```python
from build123d import *

# Parameters (mm, degrees)
F1_DEPTH    = 3
F3_DEPTH    = 5
F5_D        = 2
F5_DEPTH    = 2.001
F6_W        = 16.9
F6_H        = 5
F6_W_2      = 5
F7_DEPTH    = 4
F8_W        = 2
F8_H        = 3
F9_DEPTH    = 2.5
F11_DEPTH   = 2
F12_R       = 2
F13_SIZE2   = 1
F13_SIZE    = 0.2679491924
F14_SIZE2   = 2
F14_SIZE    = 0.5358983849
F14_2_SIZE2 = 2
F14_2_SIZE  = 0.5358983849
F15_SIZE2   = 1
F15_SIZE    = 0.5773502692
F16_W       = 15
F16_H       = 14
F17_DEPTH   = 8
F19_DEPTH   = 6
F21_D       = 2.5
F21_DEPTH   = 7.5
F21_TIP     = 0.7510757738


with BuildPart() as f1:
    # F0 (on Top) → F1 (new body, symmetric)
    with BuildSketch(Plane.XY):
        Polygon((19.45, 10), (0, 10), (-19.45, 10), (-19.45, -10), (19.45, -10), align=None)
    extrude(amount=F1_DEPTH, both=True)

    # F2 (on Front) → F3 (join, symmetric)
    with BuildSketch(Plane.XZ):
        Polygon((-8.45, 3.5893841543), (-16.45, 5), (-19.45, 5), (-19.45, 3), (-8.45, 3), align=None)
    extrude(amount=F3_DEPTH, both=True)

    # F5 (through all, one way)
    with BuildSketch(Plane(origin=(0, 0, 3), x_dir=(1, 0, 0), z_dir=(0, 0, -1))):
        with Locations((-8.45, -4), (-8.45, 4)):
            Circle(F5_D / 2)
    extrude(amount=-F5_DEPTH, mode=Mode.SUBTRACT)

    # F6 (on face) → F7 (join)
    with BuildSketch(Plane.XY.offset(3)):
        with Locations((-11, -7.5)):
            Rectangle(F6_W, F6_H)
        with Locations((-11, 7.5)):
            Rectangle(F6_W, F6_H)
        with Locations((16.95, 7.5)):
            Rectangle(F6_W_2, F6_H)
        with Locations((16.95, -7.5)):
            Rectangle(F6_W_2, F6_H)
    extrude(amount=F7_DEPTH)

    # F8 (on face) → F9 (join)
    with BuildSketch(Plane.XY.offset(3)):
        with Locations((3.45, 6.5)):
            Rectangle(F8_W, F8_H)
        with Locations((3.45, -6.5)):
            Rectangle(F8_W, F8_H)
    extrude(amount=F9_DEPTH)

    # F10 (on face) → F11 (join)
    with BuildSketch(Plane.XY.offset(3)):
        Polygon((19.45, -5), (19.45, 5), (14.45, 5), (14.45, 2), (8.45, 2), (8.45, -2), (14.45, -2), (14.45, -5), align=None)
    extrude(amount=F11_DEPTH)

    # F12
    f12_edges = [f1.edges().sort_by_distance(p)[0] for p in [
        (14.45, -2, 4),
        (14.45, 2, 4),
    ]]
    fillet(f12_edges, radius=F12_R)

    # F13
    f13_edges = [f1.edges().sort_by_distance(p)[0] for p in [
        (8.45, 0, 5),
    ]]
    f13_side = f1.faces().sort_by_distance((15.139847, 0, 5))[0]
    chamfer(f13_edges, length=F13_SIZE, length2=F13_SIZE2, reference=f13_side)

    # F14
    f14_edges = [f1.edges().sort_by_distance(p)[0] for p in [
        (-11, 5, 7),
    ]]
    f14_side = f1.faces().sort_by_distance((-11, 7.5, 7))[0]
    chamfer(f14_edges, length=F14_SIZE, length2=F14_SIZE2, reference=f14_side)

    # F14#2
    f14_2_edges = [f1.edges().sort_by_distance(p)[0] for p in [
        (-11, -5, 7),
    ]]
    f14_2_side = f1.faces().sort_by_distance((-11, -7.5, 7))[0]
    chamfer(f14_2_edges, length=F14_2_SIZE, length2=F14_2_SIZE2, reference=f14_2_side)

    # F15
    f15_edges = [f1.edges().sort_by_distance(p)[0] for p in [
        (19.45, 5, 6),
        (19.45, -5, 6),
    ]]
    f15_side = f1.faces().sort_by_distance((19.45, 0, 1.555556))[0]
    chamfer(f15_edges, length=F15_SIZE, length2=F15_SIZE2, reference=f15_side)

    # F16 (on face) → F17 (join)
    with BuildSketch(Plane(origin=(0, 0, -3), x_dir=(1, 0, 0), z_dir=(0, 0, -1))):
        Rectangle(F16_W, F16_H)
    extrude(amount=F17_DEPTH)

    # F18 (on face) → F19 (cut)
    with BuildSketch(Plane(origin=(0, 0, -11), x_dir=(1, 0, 0), z_dir=(0, 0, -1))):
        with BuildLine():
            Line((-2, 0), (-2, -1.5))
            ThreePointArc((-2, -1.5), (2.5, 0), (-2, 1.5))
            Line((-2, 1.5), (-2, 0))
        make_face()
    extrude(amount=-F19_DEPTH, mode=Mode.SUBTRACT)

    # F21
    with Locations(Plane(origin=(-7.5, 0, 0), x_dir=(0, -1, 0), z_dir=(-1, 0, 0))):
        with Locations((0, -8)):
            Hole(F21_D / 2, depth=F21_DEPTH)
            with Locations((0, 0, -(F21_DEPTH + F21_TIP / 2))):  # 118° drill point
                Cone(0, F21_D / 2, F21_TIP, mode=Mode.SUBTRACT)


solid = f1.part
```
Geometry check sheet. Reference: the model listing, model coordinates, mm. A direction names the side the tool comes from. Round coordinates to 2 decimals unless told otherwise and drop trailing zeros. Loops run counter-clockwise (first coordinate to the right, second up) from the corner with the lowest first, then second, coordinate; pieces in that order, holes last. Notation, with made-up numbers: M -27.5,78.25 L -18.5,78.25 A19 ccw -18.5,114.25 Z; hole C 76,4 d6. An arc over 180 degrees is marked long. Return JSON: item names as keys, results as strings. Group by question number.
(1) Set-up check for faces 1 (the face through (2.5, 0.1, -8)), 2 (the face through (-8, 5, 4)), 3 (the face through (10, -2, 4)): record each of +Z, -Z, +X, -X, +Y, -Y from which the full face is reachable in a straight line by a thin tool's end or side.
(2) Section check C-C, the plane x = 0. Enter the section's corners in (y, z).
(3) Section check A-A, the plane y = 0. Enter the section's corners in (x, z).
(4) Section check D-D, the plane y = -8.5. Enter the section's corners in (x, z), and give its area (3 significant figures).
(5) Go/stop test with flat-tipped pins: pin 1 (1.6 mm diameter, centred on x = 3, z = 4, fed in from -Y); pin 2 (12 mm diameter, centred on x = -12, y = -5.5, fed in from -Z); pin 3 (2 mm diameter, centred on x = -9, y = -2, fed in from +Z); pin 4 (2.5 mm diameter, centred on y = -0.5, z = -7, fed in from +X). Record where each tip stops, or that it passes through.
(6) Mould release check, pull along X, two halves, no side actions. Record for faces 4 (the face through (-19.45, 0, 2)), 5 (the face through (4.45, 6, 4)), 6 (the face through (15, 0, 5)): pulls with the +X half, pulls with the -X half, needs draft (parallel to the pull), parting line crosses it, or undercut.
(7) Section check B-B, the plane z = -8. Enter the section's corners in (x, y), and give its area (3 significant figures).
(8) Scan lines: line 1 along Y through (x, z) = (-1.5, -7.25); line 2 along X through (y, z) = (-6.5, 4.5); line 3 along Y through (x, z) = (0, -8.4). Record each from-to range of solid material in increasing order. Write a range as [from, to].
Data:
{
 "1": {"face 1": "-Z", "face 2": "+Z", "face 3": "+Z, -Y"},
 "2": {"outline": "M -10,-3 L -7,-3 L -7,-11 L -2.5,-11 L -2.5,-5 L 2.5,-5 L 2.5,-11 L 7,-11 L 7,-3 L 10,-3 L 10,3 L -10,3 Z"},
 "3": {"outline": "M -19.45,-3 L -7.5,-3 L -7.5,-6.75 L -2,-6.75 L -2,-5 L 2.5,-5 L 2.5,-11 L 7.5,-11 L 7.5,-3 L 19.45,-3 L 19.45,5 L 8.72,5 L 8.45,4 L 8.45,3 L -8.45,3 L -8.45,3.59 L -16.45,5 L -19.45,5 Z; M -7.5,-11 L -2,-11 L -2,-9.25 L -7.5,-9.25 Z"},
 "4": {"outline": "M -19.45,-3 L 19.45,-3 L 19.45,7 L 14.45,7 L 14.45,3 L -2.55,3 L -2.55,7 L -19.45,7 Z", "area": "321 mm²"},
 "5": {"pin 1": "y = -8", "pin 2": "z = -11", "pin 3": "z = 3.86", "pin 4": "x = 7.5"},
 "6": {"face 4": "pulls with the -X half", "face 5": "undercut", "face 6": "needs draft"},
 "7": {"outline": "M -7.5,-7 L 7.5,-7 L 7.5,7 L -7.5,7 L -7.5,1.25 L -2,1.25 L -2,1.5 A2.5 cw long -2,-1.5 L -2,-1.25 L -7.5,-1.25 Z", "area": "178 mm²"},
 "8": {"line 1": "[-7, -2], [2, 7]", "line 2": "[-19.45, -2.55], [2.45, 4.45], [14.45, 19.45]", "line 3": "[-7, -2.5], [2.5, 7]"}
}
